Here's how the part is built. I have some questions about the finished solid (model axes, mm). Face numbers are marked on the shaded views. A direction names the side the tool comes from. Round coordinates to 2 decimals unless told otherwise and drop trailing zeros. Write each loop counter-clockwise with the first axis right and the second up, starting at its lowest first coordinate (ties: lowest second). Pieces come first, ordered by that corner, then holes. Notation, with made-up numbers: (-20.5, 2) -> (24.5, 2) arc R21 cw to (24.5, 40) -> close; hole circle Ø2 at (7, -3). An arc over 180 degrees is marked (long way). Put each result on its own line as item: value. Start each with the question number.
1. I need wall thicknesses on probe 1 along Z at (x, y) = (-9, 8); probe 2 along X at (y, z) = (-10, 26); probe 3 along X at (y, z) = (3, 17). Which ranges of each line are inside material? Lowest first, please. Write a range as from..to.
2. We'd pull the mould along Y, two halves only. Please class the marked faces 3, 4, 5 and 6: +Y half, -Y half, draft (parallel to the pull), parting line (faces both ways), or undercut.
3. Suppose I cut it at C-C (z = 29). Please give me the cut outline in (x, y), then the cut area to 3 significant figures.
4. For pin 1 (12 mm diameter, centred on x = -32.5, z = 12.5, fed in from -Y); pin 2 (6 mm diameter, centred on y = -8, z = 21, fed in from -X); pin 3 (4 mm diameter, centred on x = -21, y = 18.5, fed in from +Z); pin 4 (14.5 mm diameter, centred on x = -45.18, y = 0, fed in from -Z), each with a flat end and sliding along its axis, tell me the tip position at first contact or that it passes through.
5. Which directions (+Z, -Z, +X, -X, +Y, -Y) give clear straight access to the entire face, cutting with the end or side of a thin tool? Please do the marked faces 1 and 2.
6. Suppose I cut it at A-A (z = 5). Please give me the cut outline in (x, y) (1 decimal), then the cut area to 3 significant figures.
7. Suppose I cut it at B-B (x = 6.5). Please give me the cut outline in (y, z).
```python
from build123d import *

# Parameters (mm, degrees)
F0_R     = 12.137084
F1_DEPTH = 41.148
F2_R     = 5.08
F0_R_2   = 7.184779
F0_R_3   = 6.643855
F3_DEPTH = 11.176
F4_R     = 12.219886


with BuildPart() as f1:
    # F0 (on Top) → F1 (new body)
    with BuildSketch(Plane.XY):
        with BuildLine():
            ThreePointArc((-26.886796, -16.617896), (-22.126002, -8.907848), (-20.464604, 0))
            ThreePointArc((-20.464604, 0), (-22.430371, 9.658588), (-28.014918, 17.780496))
            ThreePointArc((-28.014918, 17.780496), (-69.87355, -0.809985), (-26.886796, -16.617896))
        make_face()
        with Locations((-45.175716, 0)):
            Circle(F0_R, mode=Mode.SUBTRACT)
    extrude(amount=F1_DEPTH)

    # F2
    f2_edges = [f1.edges().sort_by_distance(p)[0] for p in [
        (-63.464637, 16.617896, 41.148),
    ]]
    fillet(f2_edges, radius=F2_R)

    # F0 (on Top) → F3 (join)
    with BuildSketch(Plane.XY):
        with BuildLine():
            ThreePointArc((-28.014918, 17.780496), (-22.430371, 9.658588), (-20.464604, 0))
            ThreePointArc((-20.464604, 0), (-22.126002, -8.907848), (-26.886796, -16.617896))
            Line((-26.886796, -16.617896), (25.309285, -29.663572))
            Line((25.309285, -29.663572), (25.309285, 35.378572))
            Line((25.309285, 35.378572), (-28.014918, 17.780496))
        make_face()
        with Locations((12.518571, -12.246429)):
            Circle(F0_R_2, mode=Mode.SUBTRACT)
        with Locations((9.525, 17.961429)):
            Circle(F0_R_3, mode=Mode.SUBTRACT)
    extrude(amount=F3_DEPTH)

    # F4
    f4_edges = [f1.edges().sort_by_distance(p)[0] for p in [
        (25.309285, -29.663572, 5.588),
        (25.309285, 35.378572, 5.588),
    ]]
    fillet(f4_edges, radius=F4_R)


solid = f1.part
```
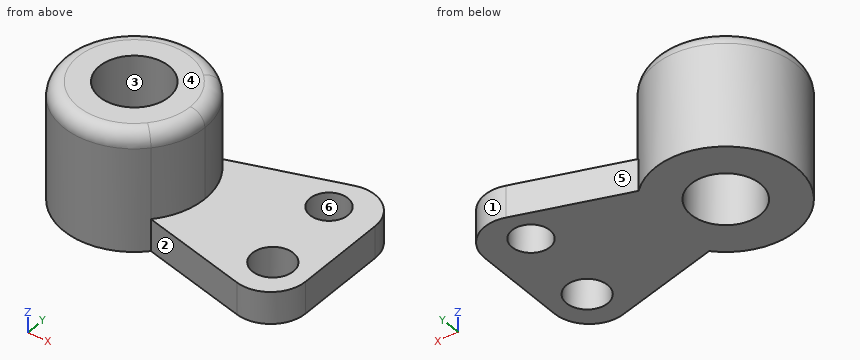
Verdict:
1. probe 1: z = 0..11.18
1. probe 2: x = -67.77..-52.05, -38.3..-22.58
1. probe 3: x = -69.7..-56.94, -33.42..-20.65
2. face 3: undercut
2. face 4: draft
2. face 5: +Y half
2. face 6: undercut
3. outline: (-26.89, -16.62) arc R24.71 ccw to (-20.46, 0) arc R24.71 ccw (long way) to start; hole circle Ø24.27 at (-45.18, 0)
3. area: 1,460 mm^2
4. pin 1: stops at y = -23.79
4. pin 2: stops at x = -69.38
4. pin 3: stops at z = 11.18
4. pin 4: passes through
5. face 1: +Z, -Z, +Y
5. face 2: +Z, -Z, -Y
6. outline: (-28, 17.8) arc R24.7 ccw (long way) to (-26.9, -16.6) -> (10.1, -25.9) arc R12.2 ccw to (25.3, -14) -> (25.3, 18.5) arc R12.2 ccw to (9.3, 30.1) -> close; hole circle Ø24.3 at (-45.2, 0); hole circle Ø13.3 at (9.5, 18); hole circle Ø14.4 at (12.5, -12.2)
6. area: 3,490 mm^2
7. outline: (-24.96, 0) -> (-16.17, 0) -> (-16.17, 11.18) -> (-24.96, 11.18) -> close; (-8.32, 0) -> (12.05, 0) -> (12.05, 11.18) -> (-8.32, 11.18) -> close; (23.88, 0) -> (29.17, 0) -> (29.17, 11.18) -> (23.88, 11.18) -> close
